Source: CAD feature listing. Evaluate the final solid. Frame: model axes, mm. Coordinates: 2 decimals unless noted, no trailing zeros. Write each loop counter-clockwise with the first axis right and the second up, starting at its lowest first coordinate (ties: lowest second). Pieces come first, ordered by that corner, then holes. Notation, with made-up numbers: M 7,-0.5 L 43,-0.5 A31 cw 43,32.5 Z; hole C -34.75,67 d7. An arc over 180 degrees is marked long. Answer as CSV lines item,"result". Start each with the question number.
1. Section A-A on x = 2. Return the cut outline in (y, z), plus the area to 3 significant figures.
2. Section D-D on x = 22. Return the cut outline in (y, z).
3. Contact query for flat-ended pins moving along their axis: pin 1 Ø12 at (x, y) = (15, 67.5) entering from -Z; pin 2 Ø4 at (x, z) = (21.5, 10) entering from +Y; pin 3 Ø1 at (x, y) = (25, 31.5) entering from +Z. Output: stop coordinate, or through.
4. Mould query, pull axis Y, two halves, no side actions, for faces 1 (the face through (14, 0, 6)), 2 (the face through (15, 35, 9.7)), 3 (the face through (20, 47, 12.7)). Classes: pulls with the +Y half, pulls with the -Y half, needs draft (parallel to the pull), parting line crosses it, or undercut.
5. Section C-C on y = 25.5. Return the cut outline in (x, z), plus the area to 3 significant figures.
6. Section B-B on z = 6.25. Return the cut outline in (x, y).
7. Line query: probe 1 along Z at (x, y) = (11.25, 23); probe 2 along Y at (x, z) = (6.75, 5.25); probe 3 along X at (y, z) = (46, 10.75). Output: solid intervals per line, ascending. Write a range as [from, to].
```python
from build123d import *

# Parameters (mm, degrees)
F1_DEPTH = 27.94
F3_DEPTH = 3
F5_DEPTH = 25.4


with BuildPart() as f1:
    # F0 (on Right) → F1 (new body)
    with BuildSketch(Plane.YZ):
        Polygon((0, 12.7), (0, 0), (50.8, 0), (76.2, 12.7), align=None)
    extrude(amount=F1_DEPTH)

    # F2 (on face) → F3 (cut)
    with BuildSketch(Plane.XY.offset(12.7)):
        with BuildLine():
            ThreePointArc((13.97, 48.006), (1.016, 35.052), (13.97, 22.098))
            Line((13.97, 22.098), (13.97, 48.006))
        make_face()
        with BuildLine():
            Line((13.97, 48.006), (13.97, 22.098))
            ThreePointArc((13.97, 22.098), (23.1298612435, 25.8921387565), (26.924, 35.052))
            ThreePointArc((26.924, 35.052), (23.1298612435, 44.2118612435), (13.97, 48.006))
        make_face()
    extrude(amount=-F3_DEPTH, mode=Mode.SUBTRACT)

    # F4 (on face) → F5 (cut)
    with BuildSketch(Plane.XY.offset(12.7)):
        with BuildLine():
            ThreePointArc((2.9316641234, 28.2725267849), (1.0181406263, 35.2874883522), (3.1854046142, 42.2282537835))
            ThreePointArc((3.1854046142, 42.2282537835), (1.6304640704, 42.7495197934), (0, 42.926))
            Line((0, 42.926), (0, 27.686))
            ThreePointArc((0, 27.686), (1.4948802796, 27.8340703329), (2.9316641234, 28.2725267849))
        make_face()
        with BuildLine():
            ThreePointArc((2.9316641234, 28.2725267849), (6.3404921189, 31.0795878466), (7.62, 35.306))
            ThreePointArc((7.62, 35.306), (6.4162755225, 39.4164511212), (3.1854046142, 42.2282537835))
            ThreePointArc((3.1854046142, 42.2282537835), (1.0181406263, 35.2874883522), (2.9316641234, 28.2725267849))
        make_face()
    extrude(amount=-F5_DEPTH, mode=Mode.SUBTRACT)


solid = f1.part
```
Values:
1,outline,"M 0,0 L 27.95,0 L 27.95,12.7 L 0,12.7 Z; M 42.66,0 L 50.8,0 L 76.2,12.7 L 42.66,12.7 Z"
1,area,"620 mm²"
2,outline,"M 0,0 L 50.8,0 L 76.2,12.7 L 45.22,12.7 L 45.22,9.7 L 24.89,9.7 L 24.89,12.7 L 0,12.7 Z"
3,pin 1,"z = 5.35"
3,pin 2,"y = 74.8"
3,pin 3,"z = 9.7"
4,face 1,"pulls with the -Y half"
4,face 2,"undercut"
4,face 3,"needs draft"
5,outline,"M 0,0 L 27.94,0 L 27.94,12.7 L 22.72,12.7 L 22.72,9.7 L 5.22,9.7 L 5.22,12.7 L 0,12.7 Z"
5,area,"302 mm²"
6,outline,"M 0,0 L 27.94,0 L 27.94,63.3 L 0,63.3 L 0,42.93 A7.62 cw 0,27.69 Z"
7,probe 1,"[0, 9.7]"
7,probe 2,"[0, 31.77], [38.84, 61.3]"
7,probe 3,"[0, 7.05], [20.89, 27.94]"
